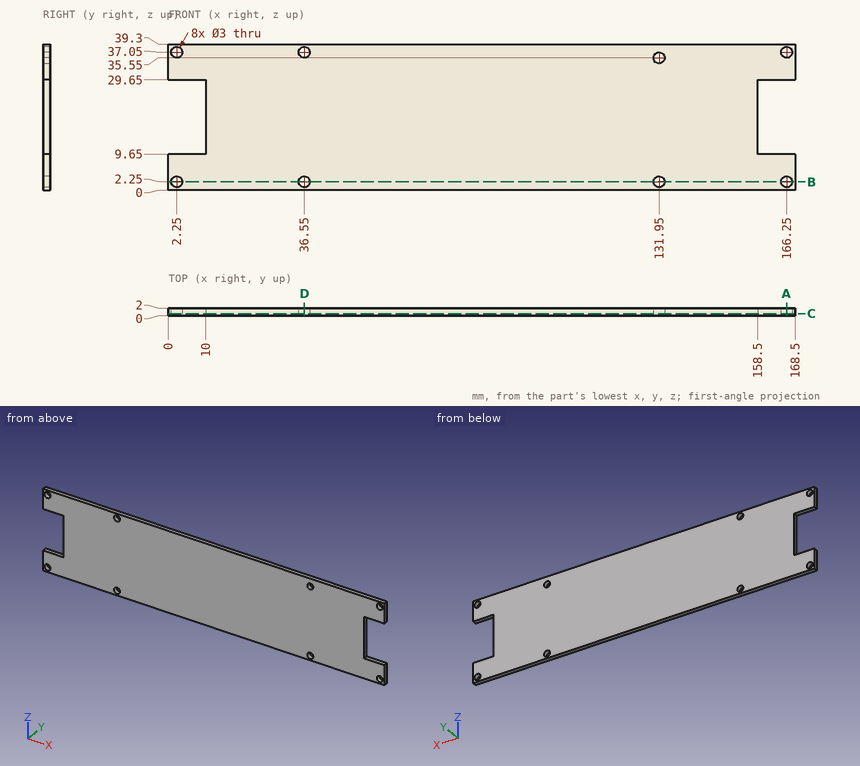
Verification items for this drawing (mm, ordinates from the low corner). Give positions to 0.01 mm unless a question says otherwise; leave off trailing zeros. Loops run counter-clockwise (first coordinate to the right, second up) from the corner with the lowest first, then second, coordinate; pieces in that order, holes last. Notation, with made-up numbers: M 27.25,63 L 35.25,63 A18 ccw 35.25,73 Z; hole C 45,76.5 d6. An arc over 180 degrees is marked long. Answer as a JSON object with one key per item and string values. Group by question number.
Q1. Material ranges on line 1 along Z through (x, y) = (166.25, 1.5); line 2 along X through (y, z) = (1.4, 2.5); line 3 along X through (y, z) = (1.2, 11.5), recorded low to high. Write a range as [from, to].
Q2. Cross-section at C-C on y = 0.5. Give the number of separate pieces and of enclosed holes in the cut face, then the cut area to 3 significant figures.
Q3. Go/stop test with a flat-tipped pin: P1, Ø1, axis at y = 1, z = 24.5, coming from the +X side. Record where the tip stops, or that it passes through.
Q4. Cross-section at A-A on x = 166.25. Record the cut outline in (y, z).
Q5. Cross-section at B-B on z = 2.25. Record the cut outline in (x, y).
Q6. Cross-section at D-D on x = 36.55. Record the cut outline in (y, z).
Evaluation:
{
 "1": {"line 1": "z = [0, 0.75], [3.75, 9.65], [29.65, 35.55], [38.55, 39.3]", "line 2": "x = [0, 0.77], [3.73, 35.07], [38.03, 130.47], [133.43, 164.77], [167.73, 168.5]", "line 3": "x = [10, 158.5]"},
 "2": {"separate pieces": "1", "enclosed holes": "8", "area": "6,170 mm2"},
 "3": {"P1": "stops at x = 158.5"},
 "4": {"outline": "M 0,0 L 2,0 L 2,0.75 L 0,0.75 Z; M 0,3.75 L 2,3.75 L 2,9.65 L 0,9.65 Z; M 0,29.65 L 2,29.65 L 2,35.55 L 0,35.55 Z; M 0,38.55 L 2,38.55 L 2,39.3 L 0,39.3 Z"},
 "5": {"outline": "M 0,0 L 0.75,0 L 0.75,2 L 0,2 Z; M 3.75,0 L 35.05,0 L 35.05,2 L 3.75,2 Z; M 38.05,0 L 130.45,0 L 130.45,2 L 38.05,2 Z; M 133.45,0 L 164.75,0 L 164.75,2 L 133.45,2 Z; M 167.75,0 L 168.5,0 L 168.5,2 L 167.75,2 Z"},
 "6": {"outline": "M 0,0 L 2,0 L 2,0.75 L 0,0.75 Z; M 0,3.75 L 2,3.75 L 2,35.55 L 0,35.55 Z; M 0,38.55 L 2,38.55 L 2,39.3 L 0,39.3 Z"}
}
